from build123d import *

# Parameters (mm, degrees)
F0_W     = 57.15
F0_H     = 19.05
F1_DEPTH = 152.4


# Not quite as in the source:
# - ends of sketch curves that miss each other by under 0.0002 mm in the source are joined


with BuildPart() as f1:
    # F0 (on Front) → F1 (new body)
    with BuildSketch(Plane.XZ):
        with BuildLine():
            Line((4.745863, -11.1335566), (4.745863, -30.1835566))
            Line((4.745863, -30.1835566), (11.100308, -30.1835566))
            ThreePointArc((11.100308, -30.1835566), (14.8226482602, -21.1970322602), (23.8091726, -17.474692))
            Line((23.8091726, -17.474692), (23.8091726, -11.120247))
            ThreePointArc((23.8091726, -11.120247), (32.8666183043, -5.8802359043), (38.1066276666, 3.1772102678))
            ThreePointArc((38.1066276666, 3.1772102678), (43.4430736289, 12.1382508388), (52.4041076698, 17.4747052267))
            Line((52.4041076698, 17.4747052267), (52.4041116, 30.1835566))
            Line((52.4041116, 30.1835566), (38.0344934, 30.1835566))
            Line((38.0344934, 30.1835566), (4.745863, -7.9430372))
            Line((4.745863, -7.9430372), (4.745863, -11.1335566))
        make_face()
        with Locations((-23.829137, -20.6585566)):
            Rectangle(F0_W, F0_H)
    extrude(amount=F1_DEPTH)


solid = f1.part
Check sheet for the modelled part. Datum: model origin and axes. Units: mm. A direction names the side the tool comes from. Round coordinates to 2 decimals unless told otherwise and drop trailing zeros. Loops run counter-clockwise (first coordinate to the right, second up) from the corner with the lowest first, then second, coordinate; pieces in that order, holes last. Notation, with made-up numbers: M 82.5,4 L 110.5,4 A10 ccw 110.5,19 Z; hole C 12.5,28.25 d10. An arc over 180 degrees is marked long. One line per item, written item: value.
(1) Sectioned sample at B-B, the plane x = -39.5. Record the cut outline in (y, z), then the cut area to 3 significant figures.
Computed values:
outline: M -152.4,-30.18 L 0,-30.18 L 0,-11.13 L -152.4,-11.13 Z
area: 2,900 mm^2
(2) Depth check by flat-ended pin: pin 1 Ø1 at (y, z) = (-136.5, 23) entering from -X; pin 2 Ø3 at (x, z) = (3.5, -13) entering from +Y; pin 3 Ø1.6 at (y, z) = (-52.5, -9) entering from -X; pin 4 Ø1 at (y, z) = (-107, 12.5) entering from +X. Enter the tip coordinate at first touch or a pass-through.
Computed values:
pin 1: stops at x = 31.33
pin 2: stops at y = 0
pin 3: stops at x = 4.75
pin 4: stops at x = 44.36
(3) Access from +Z, -Z, +X, -X, +Y, -Y to the whole of each face (thin tool, end or side, straight path). Record for faces 1 (the face through (23.809, -75, -14)), 2 (the face through (8, 0, -9)), 3 (the face through (4.746, -75, -10)).
Computed values:
face 1: -Z, +X, +Y, -Y
face 2: +Z, -Z, +X, -X, +Y
face 3: +Z, -X, +Y, -Y
(4) Sectioned sample at A-A, the plane y = -83.5. Record the cut outline in (x, z).
Computed values:
outline: M -52.4,-30.18 L 11.1,-30.18 A12.71 cw 23.81,-17.47 L 23.81,-11.12 A20.28 ccw 38.11,3.18 A21.22 cw 52.4,17.47 L 52.4,30.18 L 38.03,30.18 L 4.75,-7.94 L 4.75,-11.13 L -52.4,-11.13 Z
(5) Sectioned sample at C-C, the plane z = 15. Record the cut outline in (x, y), then the cut area to 3 significant figures.
Computed values:
outline: M 24.78,-152.4 L 47,-152.4 L 47,0 L 24.78,0 Z
area: 3,390 mm^2
(6) Thickness scan on line 1 (Z direction, x = -35.5, y = -80.5); line 2 (X direction, y = -95, z = -13.5); line 3 (X direction, y = -120.5, z = 19). Record the ranges inside material, lowest first.
Computed values:
line 1: z = -30.18 to -11.13
line 2: x = -52.4 to 23.81
line 3: x = 28.27 to 52.4
